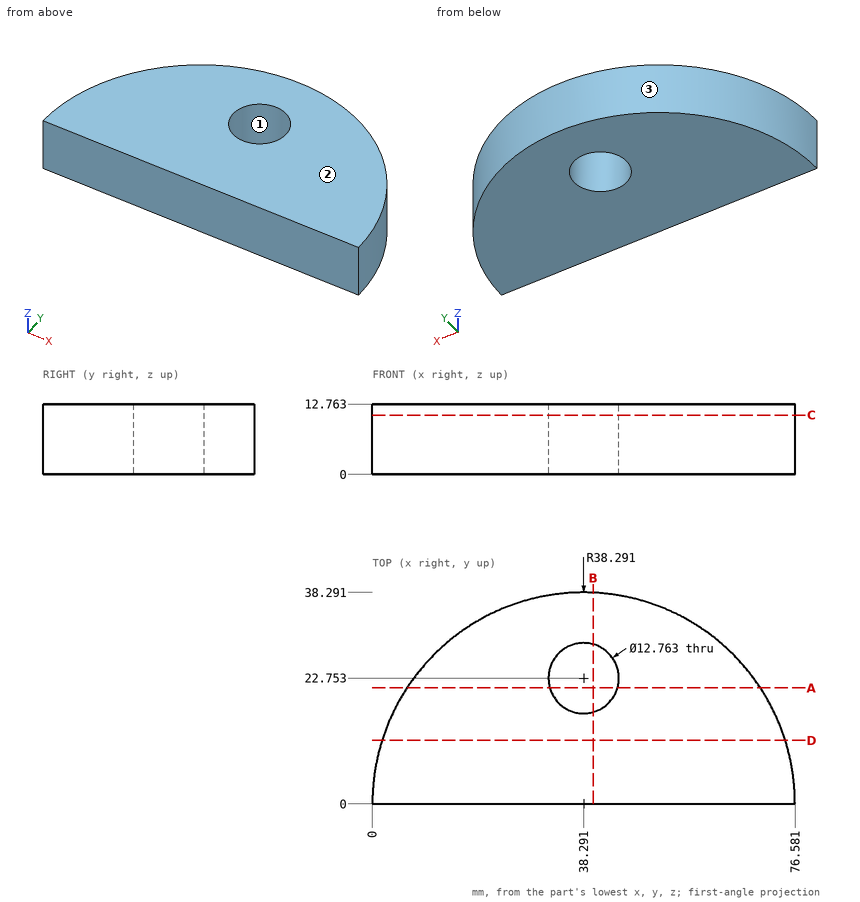
Answer from the drawing. Dimensions are ordinates in mm from the lowest x, y and z of the part. Coordinates: 2 decimals unless noted, no trailing zeros. Loops run counter-clockwise (first coordinate to the right, second up) from the corner with the lowest first, then second, coordinate; pieces in that order, holes last. Notation, with made-up numbers: (61.5, -10) - (65.5, -10) arc R8 ccw to (65.5, 4) - close; hole circle Ø9 at (34, 44). An arc over 180 degrees is marked (long way). Answer in a Markdown table with one row per item.
1. Given pin 1 (3 mm diameter, centred on y = 32, z = 6, fed in from +X); pin 2 (4 mm diameter, centred on x = 54.5, z = 9, fed in from +Y), each flat-ended and moving along its own axis, determine where each tip first touches the part or whether it passes through.
Conclusion:
| item | result |
|---|---|
| pin 1 | stops at x = 61.44 |
| pin 2 | stops at y = 35.56 |
2. Find section A-A, the plane y = 21. Write down the section's boundary in (x, z) (1 decimal).
Conclusion:
| item | result |
|---|---|
| outline | (6.3, 0) - (32.2, 0) - (32.2, 12.8) - (6.3, 12.8) - close; (44.4, 0) - (70.3, 0) - (70.3, 12.8) - (44.4, 12.8) - close |
3. Straight lines are drawn through the part: line 1 (X direction, y = 28.5, z = 10.5) (1 decimal); line 2 (X direction, y = 22.5, z = 10) (1 decimal); line 3 (Y direction, x = 55, z = 5). For each, find the intervals that lie inside material, in ascending order.
Conclusion:
| item | result |
|---|---|
| line 1 | x = 12.7 to 35.5, 41.1 to 63.9 |
| line 2 | x = 7.3 to 31.9, 44.7 to 69.3 |
| line 3 | y = 0 to 34.45 |
4. Find section B-B, the plane x = 40. Write down the section's boundary in (y, z) (1 decimal).
Conclusion:
| item | result |
|---|---|
| outline | (0, 0) - (16.6, 0) - (16.6, 12.8) - (0, 12.8) - close; (28.9, 0) - (38.3, 0) - (38.3, 12.8) - (28.9, 12.8) - close |
5. Find section C-C, the plane z = 10.75. Write down the section's boundary in (x, y).
Conclusion:
| item | result |
|---|---|
| outline | (0, 0) - (76.58, 0) arc R38.29 ccw to start; hole circle Ø12.76 at (38.29, 22.75) |
6. Determine the mould class of the marked faces 1, 2 and 3 for opening direction X: +X half, -X half, draft (parallel to the pull), parting line (faces both ways), or undercut.
Conclusion:
| item | result |
|---|---|
| face 1 | undercut |
| face 2 | draft |
| face 3 | parting line |
7. Find section D-D, the plane y = 11.5. Write down the section's boundary in (x, z), then the cut area to 3 significant figures.
Conclusion:
| item | result |
|---|---|
| outline | (1.77, 0) - (74.81, 0) - (74.81, 12.76) - (1.77, 12.76) - close |
| area | 932 mm² |
